Input: part model. Units: mm. Frame: model coordinates. Face numbers are marked on the shaded views. Give positions to 0.01 mm unless a question says otherwise; leave off trailing zeros. Loops run counter-clockwise (first coordinate to the right, second up) from the corner with the lowest first, then second, coordinate; pieces in that order, holes last.
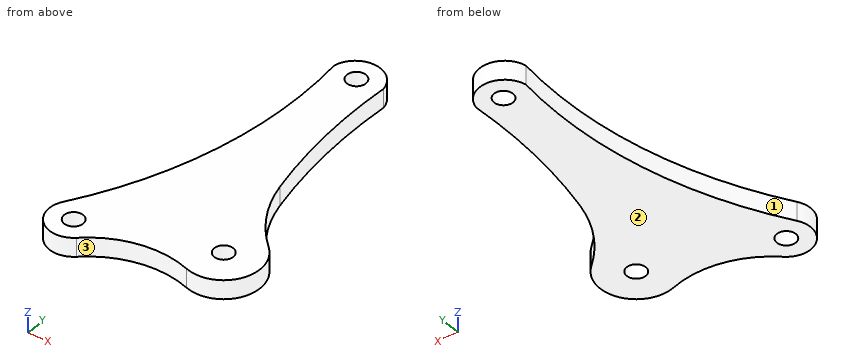
from build123d import *

# Parameters (mm, degrees)
ESQUISSE1_R               = 1.5
T_LE_DE_BASE_PLI_E1_DEPTH = 3


# Sheet-metal steps are written as plain solids
with BuildPart() as part:
    # Esquisse1 → Tôle de base pliée1 (new body)
    with BuildSketch(Plane.XY):
        with BuildLine():
            ThreePointArc((1266.925045451, 1453.637099805), (1270.853858472, 1456.885815408), (1274.782671493, 1453.637099805))
            ThreePointArc((1274.782671493, 1453.637099805), (1274.958888422, 1441.583989625), (1276.882340742, 1429.684038004))
            ThreePointArc((1276.882340742, 1429.684038004), (1279.307388945, 1423.763410381), (1283.429682965, 1418.870417202))
            ThreePointArc((1283.429682965, 1418.870417202), (1284.686333081, 1411.736203474), (1277.965134068, 1409.03404529))
            ThreePointArc((1277.965134068, 1409.03404529), (1270.106079959, 1409.318689972), (1263.166360558, 1405.619223969))
            ThreePointArc((1263.166360558, 1405.619223969), (1258.081900759, 1405.461151241), (1257.278806491, 1410.484273581))
            ThreePointArc((1257.278806491, 1410.484273581), (1265.841325108, 1431.224793872), (1266.925045451, 1453.637099805))
        make_face()
        with Locations((1279.65990658, 1414.528610435)):
            Circle(ESQUISSE1_R, mode=Mode.SUBTRACT)
        with Locations((1260.534319165, 1408.429002982)):
            Circle(ESQUISSE1_R, mode=Mode.SUBTRACT)
        with Locations((1270.855299475, 1453.137882296)):
            Circle(ESQUISSE1_R, mode=Mode.SUBTRACT)
    extrude(amount=-T_LE_DE_BASE_PLI_E1_DEPTH)


solid = part.part
(1) Pin query (flat end, axial travel): pin 1 Ø8 at (x, y) = (1281.5, 1448) entering from +Z; pin 2 Ø1.5 at (y, z) = (1435.5, -2.5) entering from -X; pin 3 Ø1.5 at (y, z) = (1411.5, -2.5) entering from -X. Return the tip coordinate at first contact, or that it passes through.
Values follow:
pin 1: passes through
pin 2: stops at x = 1266.53
pin 3: stops at x = 1257.45
(2) Ray query, probe 1 along Y at (x, z) = (1260.5, -0.95); probe 2 along Y at (x, z) = (1270.25, -2.45); probe 3 along X at (y, z) = (1415, -1.05). Return the intervals inside material, ascending.
Values follow:
probe 1: y = 1404.58 to 1406.93, 1409.93 to 1416.2
probe 2: y = 1409.35 to 1451.77, 1454.51 to 1456.84
probe 3: x = 1259.89 to 1278.24, 1281.08 to 1285.39
(3) Cut plane B-B (y = 1421.5). Return the cut outline in (x, z).
Values follow:
outline: (1262.86, -3) - (1280.89, -3) - (1280.89, 0) - (1262.86, 0) - close
(4) Cut plane C-C (x = 1273.75). Return the cut outline in (y, z), and give its area (3 significant figures).
Values follow:
outline: (1409.7, -3) - (1455.64, -3) - (1455.64, 0) - (1409.7, 0) - close
area: 138 mm2
(5) Cut plane A-A (z = -1.55). Return the cut outline in (x, y).
Values follow:
outline: (1257.28, 1410.48) arc R3.85 ccw to (1263.17, 1405.62) arc R15.13 cw to (1277.97, 1409.03) arc R5.75 ccw to (1283.43, 1418.87) arc R20.63 cw to (1276.88, 1429.68) arc R82.85 cw to (1274.78, 1453.64) arc R4 ccw to (1266.93, 1453.64) arc R65.7 cw to start; hole circle Ø3 at (1260.53, 1408.43); hole circle Ø3 at (1270.86, 1453.14); hole circle Ø3 at (1279.66, 1414.53)
(6) Mould query, pull axis X, two halves, no side actions, for the marked faces 1, 2 and 3. Classes: +X half, -X half, draft (parallel to the pull), parting line (faces both ways), or undercut.
Values follow:
face 1: -X half
face 2: draft
face 3: undercut
